Geometry check sheet. Reference: the model listing, model coordinates, mm. A direction names the side the tool comes from. Give positions to 0.01 mm unless a question says otherwise; leave off trailing zeros. Write each loop counter-clockwise with the first axis right and the second up, starting at its lowest first coordinate (ties: lowest second). Pieces come first, ordered by that corner, then holes. Notation, with made-up numbers: (12, 46.5) -> (55, 46.5) arc R13 ccw to (55, 57.5) -> close; hole circle Ø1 at (5, 48.5). An arc over 180 degrees is marked (long way). Write item = value, one per line. Start each with the question number.
1. Cross-section at B-B, the plane x = 0. Record the cut outline in (y, z).
2. Set-up check for faces 1 (the flat face through (-1, -41, 70)), 2 (the flat face through (100, -40, 1)): record each of +Z, -Z, +X, -X, +Y, -Y from which the full face is reachable in a straight line by a thin tool's end or side.
3. Cross-section at D-D, the plane z = 5. Record the cut outline in (x, y).
4. Thickness scan on line 1 along X through (y, z) = (-47.5, -65); line 2 along Z through (x, y) = (57, -64); line 3 along X through (y, z) = (2.85, -30). Record the ranges inside material, lowest first.
5. Mould release check, pull along Z, two halves, no side actions. Record for faces 3 (the flat face through (-1, -39, 75)), 4 (the cylindrical face through (-98.797, -40.067, -73.859)), 5 (the cylindrical face through (1.302, -1.203, -68.859)): pulls with the +Z half, pulls with the -Z half, needs draft (parallel to the pull), parting line crosses it, or undercut.
6. Cross-section at C-C, the plane y = -22.5. Record the cut outline in (x, z), plus the area to 3 significant figures.
7. Depth check by flat-ended pin: P1, Ø18, axis at x = -65, z = 30, coming from the +Y side. Enter the tip coordinate at first touch or a pass-through.
8. Cross-section at A-A, the plane z = -30. Record the cut outline in (x, y).
```python
from build123d import *

# Parameters (mm, degrees)
ESBO_O1_W                = 200
ESBO_O1_H                = 150
RESSALTO_EXTRUS_O1_DEPTH = 5
ESBO_O2_W                = 3
ESBO_O2_H                = 150
RESSALTO_EXTRUS_O2_DEPTH = 80
ESBO_O3_R                = 11.25
CORTE_EXTRUS_O1_DEPTH    = 5
ESBO_O6_W                = 194
ESBO_O6_H                = 5
RESSALTO_EXTRUS_O3_DEPTH = 80
FILETE2_R                = 4
FILETE3_R                = 4
ESBO_O12_R               = 14.229327837
CORTE_EXTRUS_O3_DEPTH    = 5


with BuildPart() as part:
    # Esboço1 → Ressalto-extrusão1 (new body)
    with BuildSketch(Plane(origin=(0, 0, 0), x_dir=(1, 0, 0), z_dir=(0, 1, 0))):
        Rectangle(ESBO_O1_W, ESBO_O1_H)
    extrude(amount=RESSALTO_EXTRUS_O1_DEPTH)

    # Esboço2 → Ressalto-extrusão2 (add)
    with BuildSketch(Plane.XZ):
        with Locations((-98.5, 0)):
            Rectangle(ESBO_O2_W, ESBO_O2_H)
        with Locations((98.5, 0)):
            Rectangle(ESBO_O2_W, ESBO_O2_H)
    extrude(amount=RESSALTO_EXTRUS_O2_DEPTH)

    # Esboço3 → Corte-extrusão1 (cut)
    with BuildSketch(Plane(origin=(0, 5, 0), x_dir=(1, 0, 0), z_dir=(0, 1, 0))):
        with Locations(Location((-65, 30, 0), (0, 0, 270))):
            Circle(ESBO_O3_R)
        with Locations(Location((-21.666666667, 30, 0), (0, 0, 270))):
            Circle(ESBO_O3_R)
        with Locations(Location((21.666666667, 30, 0), (0, 0, 270))):
            Circle(ESBO_O3_R)
        with Locations(Location((65, 30, 0), (0, 0, 270))):
            Circle(ESBO_O3_R)
        with Locations(Location((-65, -30, 0), (0, 0, 270))):
            Circle(ESBO_O3_R)
        with Locations(Location((0, -30, 0), (0, 0, 270))):
            Circle(ESBO_O3_R)
        with Locations(Location((65, -30, 0), (0, 0, 270))):
            Circle(ESBO_O3_R)
    extrude(amount=-CORTE_EXTRUS_O1_DEPTH, mode=Mode.SUBTRACT)

    # Esboço6 → Ressalto-extrusão3 (add)
    with BuildSketch(Plane.XZ):
        with Locations((0, -72.5)):
            Rectangle(ESBO_O6_W, ESBO_O6_H)
        with Locations((0, 72.5)):
            Rectangle(ESBO_O6_W, ESBO_O6_H)
    extrude(amount=RESSALTO_EXTRUS_O3_DEPTH)

    # Filete2
    filete2_edges = [part.edges().sort_by_distance(p)[0] for p in [
        (100, 5, 0),
        (0, 5, -75),
        (-100, 5, 0),
        (-100, -37.5, -75),
        (100, -37.5, -75),
        (100, -37.5, 75),
        (-100, -37.5, 75),
        (0, 5, 75),
    ]]
    fillet(filete2_edges, radius=FILETE2_R)

    # Filete3
    filete3_edges = [part.edges().sort_by_distance(p)[0] for p in [
        (-97, 0, 0),
        (97, 0, 0),
        (-97, -40, -70),
        (0, 0, -70),
        (97, -40, -70),
        (0, 0, 70),
        (-97, -40, 70),
        (97, -40, 70),
    ]]
    fillet(filete3_edges, radius=FILETE3_R)

    # Esboço12 → Corte-extrusão3 (cut)
    with BuildSketch(Plane(origin=(0, 0, -75), x_dir=(-1, 0, 0), z_dir=(0, 0, -1))):
        with Locations((0, -55.444674629)):
            Circle(ESBO_O12_R)
    extrude(amount=-CORTE_EXTRUS_O3_DEPTH, mode=Mode.SUBTRACT)


solid = part.part
```
Answers:
q1.outline = (-80, -75) -> (-69.67, -75) -> (-69.67, -70) -> (-80, -70) -> close; (-80, 70) -> (-4, 70) arc R4 cw to (0, 66) -> (0, 41.25) -> (5, 41.25) -> (5, 71) arc R4 ccw to (1, 75) -> (-80, 75) -> close; (-41.22, -75) -> (1, -75) arc R4 ccw to (5, -71) -> (5, 18.75) -> (0, 18.75) -> (0, -66) arc R4 cw to (-4, -70) -> (-41.22, -70) -> close
q2.face_1 = -Y
q2.face_2 = +Z, -Z, +X, +Y, -Y
q3.outline = (-100, -80) -> (-97, -80) -> (-97, -4) arc R4 cw to (-93, 0) -> (93, 0) arc R4 cw to (97, -4) -> (97, -80) -> (100, -80) -> (100, 1) arc R4 ccw to (96, 5) -> (-96, 5) arc R4 ccw to (-100, 1) -> close
q4.line_1 = -100 to -97, 97 to 100
q4.line_2 = -75 to -70, 70 to 75
q4.line_3 = -99.55 to -76.25, -53.75 to -32.92, -10.42 to 10.42, 32.92 to 53.75, 76.25 to 99.55
q5.face_3 = pulls with the +Z half
q5.face_4 = pulls with the -Z half
q5.face_5 = undercut
q6.outline = (-100, -71) arc R4 ccw to (-96, -75) -> (96, -75) arc R4 ccw to (100, -71) -> (100, 71) arc R4 ccw to (96, 75) -> (-96, 75) arc R4 ccw to (-100, 71) -> close; hole (-97, -66) arc R4 ccw to (-93, -70) -> (93, -70) arc R4 ccw to (97, -66) -> (97, 66) arc R4 ccw to (93, 70) -> (-93, 70) arc R4 ccw to (-97, 66) -> close
q6.area = 2,840 mm^2
q7.P1 = through
q8.outline = (-100, -80) -> (-97, -80) -> (-97, -4) arc R4 cw to (-93, 0) -> (-76.25, 0) -> (-76.25, 5) -> (-96, 5) arc R4 ccw to (-100, 1) -> close; (-53.75, 0) -> (-32.92, 0) -> (-32.92, 5) -> (-53.75, 5) -> close; (-10.42, 0) -> (10.42, 0) -> (10.42, 5) -> (-10.42, 5) -> close; (32.92, 0) -> (53.75, 0) -> (53.75, 5) -> (32.92, 5) -> close; (76.25, 0) -> (93, 0) arc R4 cw to (97, -4) -> (97, -80) -> (100, -80) -> (100, 1) arc R4 ccw to (96, 5) -> (76.25, 5) -> close
